```python
from build123d import *

# Parameters (mm, degrees)
F0_R     = 1.5875
F1_DEPTH = 1.5875
F2_SIZE  = 0.508


with BuildPart() as f1:
    # F0 (on Front) → F1 (new body, symmetric)
    with BuildSketch(Plane.XZ):
        with BuildLine():
            Line((6.503597, 2.54), (-5.810977, 2.54))
            ThreePointArc((-5.810977, 2.54), (-6.314305, 0), (-5.810977, -2.54))
            Line((-5.810977, -2.54), (5.106739, -2.54))
            Line((5.106739, -2.54), (6.503597, 2.54))
        make_face()
        with Locations((0.34631, 0)):
            Circle(F0_R, mode=Mode.SUBTRACT)
    extrude(amount=F1_DEPTH, both=True)

    # F2
    f2_edges = [f1.edges().sort_by_distance(p)[0] for p in [
        (6.503597, 0, 2.54),
    ]]
    chamfer(f2_edges, length=F2_SIZE)


solid = f1.part
```
Can you work these out from the model? Positions are in its coordinate system, mm. Round coordinates to 2 decimals unless told otherwise and drop trailing zeros. Loops run counter-clockwise (first coordinate to the right, second up) from the corner with the lowest first, then second, coordinate; pieces in that order, holes last.
Item 1: Suppose I cut it at C-C, the plane y = -0.1. Write out the boundary of the cut face in (x, z) (1 decimal), then the cut area to 3 significant figures.
Item 2: Will this pin go through, and if not, where does the flat tip stop? pin 1 Ø3 at (x, z) = (0.35, 0) entering from +Y.
Item 3: Suppose I cut it at A-A, the plane x = -1. Write out the boundary of the cut face in (y, z), then the cut area to 3 significant figures.
Item 4: Suppose I cut it at B-B, the plane z = -1.1. Write out the boundary of the cut face in (x, y), then the cut area to 3 significant figures.
Item 5: Please list where these lines run through material, in increasing order: L1, parallel to Z at x = 1.25, y = 0.4; L2, parallel to Z at x = 0.75, y = 0.9; L3, parallel to X at y = -0.9, z = 1.05.
Item 6: If we mould it in two halves opening along X, with no side actions, what happens to faces 1 (the cylindrical face through (-6.314, -0.022, 0.036)), 2 (the flat face through (5.73, -0.02, -0.28)), 3 (the flat face through (-1.5, 1.588, 0)), 4 (the cylindrical face through (1.08, 0.02, -1.41))? For each: +X half, -X half, draft (parallel to the pull), parting line (faces both ways), or undercut.
Item 7: Suppose I cut it at D-D, the plane z = -1.85. Write out the boundary of the cut face in (x, y).
Reported:
1. outline: (-5.8, -2.5) - (5.1, -2.5) - (6.4, 2.1) - (6, 2.5) - (-5.8, 2.5) arc R6.7 ccw to start; hole circle Ø3.2 at (0.3, 0)
1. area: 52.7 mm2
2. pin 1: passes through
3. outline: (-1.59, -2.54) - (1.59, -2.54) - (1.59, -0.84) - (-1.59, -0.84) - close; (-1.59, 0.84) - (1.59, 0.84) - (1.59, 2.54) - (-1.59, 2.54) - close
3. area: 10.8 mm2
4. outline: (-6.22, -1.59) - (-0.8, -1.59) - (-0.8, 1.59) - (-6.22, 1.59) - close; (1.49, -1.59) - (5.5, -1.59) - (5.5, 1.59) - (1.49, 1.59) - close
4. area: 30.0 mm2
5. L1: z = -2.54 to -1.31, 1.31 to 2.54
5. L2: z = -2.54 to -1.54, 1.54 to 2.54
5. L3: x = -6.23 to -0.84, 1.54 to 6.09
6. face 1: -X half
6. face 2: +X half
6. face 3: draft
6. face 4: undercut
7. outline: (-6.05, -1.59) - (5.3, -1.59) - (5.3, 1.59) - (-6.05, 1.59) - close
